Print and shaded views of the part. All mm, measured from the part's lowest x, y and z. A direction names the side the tool comes from. Coordinates: 2 decimals unless noted, no trailing zeros. Order: outer loops, then holes, each group sorted by start corner. A loop starts at its lowest first (then second) coordinate and runs counter-clockwise, first axis right, second up. Notation, with made-up numbers: M 24,71.5 L 82,71.5 A29 ccw 82,91.5 Z; hole C -18.5,12 d6. An arc over 180 degrees is marked long. One line per item, written item: value.
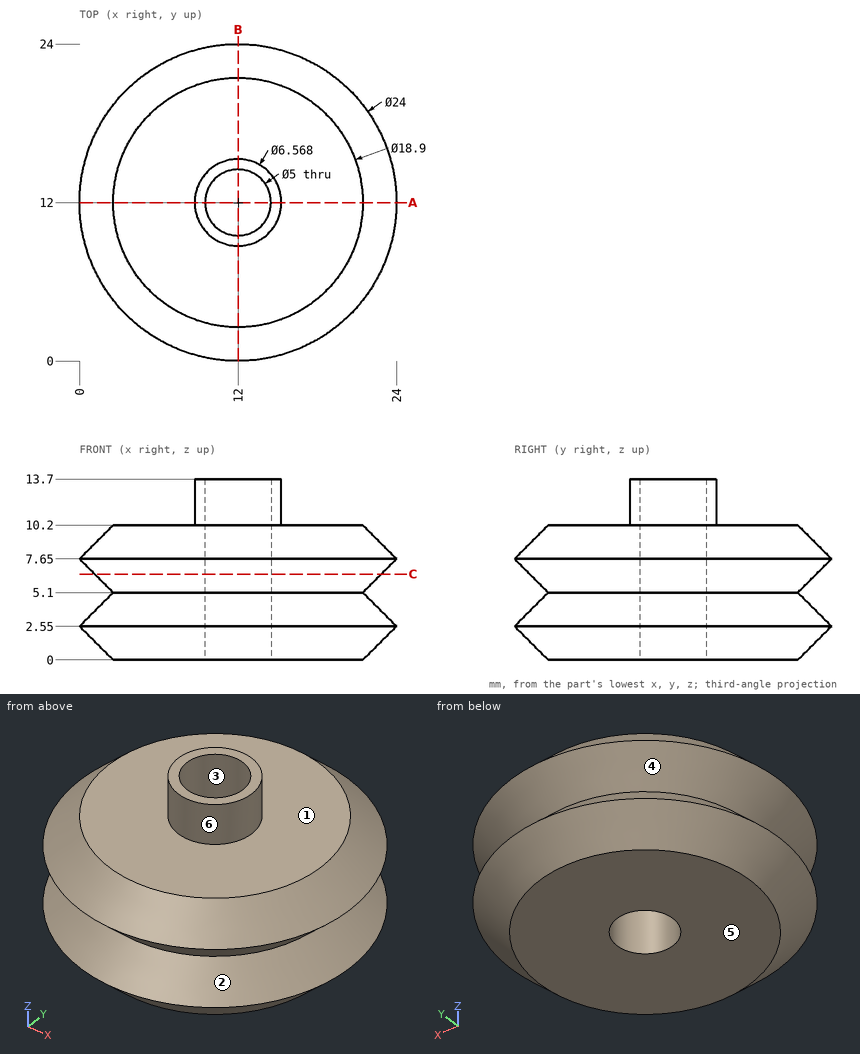
Q1. Pin check, flat tips, straight feed: pin 1 Ø4 at (x, z) = (7.5, 4.5) entering from -Y; pin 2 Ø4 at (x, y) = (11, 10) entering from +Z; pin 3 Ø6 at (y, z) = (9.5, 11) entering from -X; pin 4 Ø8 at (x, y) = (7.5, 3.5) entering from +Z. Stop position of each tip, or through.
Recorded:
pin 1: stops at y = 0.7
pin 2: stops at z = 13.7
pin 3: stops at x = 0.57
pin 4: stops at z = 10.2
Q2. Slice it at A-A (y = 12). List the corners of the cut face in (x, z), plus the area to 3 significant figures.
Recorded:
outline: M 0,2.55 L 2.55,0 L 9.5,0 L 9.5,13.7 L 8.72,13.7 L 8.72,10.2 L 2.55,10.2 L 0,7.65 L 2.55,5.1 Z; M 14.5,0 L 21.45,0 L 24,2.55 L 21.45,5.1 L 24,7.65 L 21.45,10.2 L 15.28,10.2 L 15.28,13.7 L 14.5,13.7 Z
area: 173 mm^2
Q3. Mould opens along Y. For the marked faces 1, 2 and 3 say: released by +Y, released by -Y, zero draft, split by the parting line, or undercut.
Recorded:
face 1: zero draft
face 2: split by the parting line
face 3: undercut
Q4. Slice it at C-C (z = 6.5). List the corners of the cut face in (x, y), plus the area to 3 significant figures.
Recorded:
outline: C 12,12 d21.7; hole C 12,12 d5
area: 350 mm^2
Q5. Which spindle directions (+Z, -Z, +X, -X, +Y, -Y) get a long thin tool onto all of the face, cutting with end or side? Do the marked faces 4, 5 and 6. Say none if no direction does.
Recorded:
face 4: none
face 5: -Z, +X, -X, +Y, -Y
face 6: +Z
Q6. Drill centre lines: line 1 along X through (y, z) = (11.5, 3.5); line 2 along Y through (x, z) = (12, 7.75); line 3 along Y through (x, z) = (12, 5.75). Where is each one in solid material? Low to high.
Recorded:
line 1: x = 0.96 to 9.55, 14.45 to 23.04
line 2: y = 0.1 to 9.5, 14.5 to 23.9
line 3: y = 1.9 to 9.5, 14.5 to 22.1
